from build123d import *

# Parameters (mm, degrees)
CHANFREIN1_SIZE = 0.5


with BuildPart() as part:
    # Esquisse1 → Révolution1 (revolve)
    with BuildSketch(Plane(origin=(0, 0, -20.980989745), x_dir=(-1, 0, 0), z_dir=(0, 0, -1)), mode=Mode.PRIVATE) as r_volution1_sk:
        Polygon((176.591924368, 38.325618202), (176.591924368, 34.825618202), (178.091924368, 34.825618202), (178.091924368, 36.825618202), (181.591924368, 36.825618202), (181.591924368, 38.325618202), align=None)
    revolve(r_volution1_sk.sketch.rotate(Axis((-182.472480167, 39.825618202, -20.980989745), (1, 0, 0)), 270), axis=Axis((-182.472480167, 39.825618202, -20.980989745), (1, 0, 0)))

    # Chanfrein1
    chanfrein1_edges = [part.edges().sort_by_distance(p)[0] for p in [
        (-181.591924368, 39.825618202, -23.980989745),
    ]]
    chamfer(chanfrein1_edges, length=CHANFREIN1_SIZE)


solid = part.part
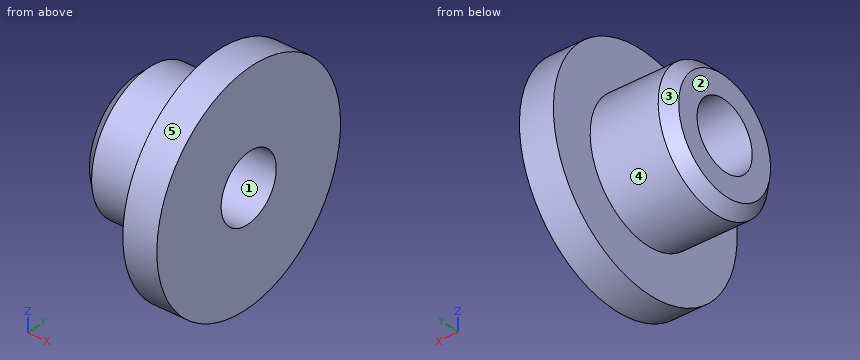
Could you check a few things on this model? Use its own coordinates, in mm. Face numbers are marked on the shaded views. A direction names the side the tool comes from. Coordinates: 2 decimals unless noted, no trailing zeros. Loops run counter-clockwise (first coordinate to the right, second up) from the corner with the lowest first, then second, coordinate; pieces in that order, holes last.
1. Imagine slicing it at A-A (z = -16.75). Please give me the cut outline in (x, y), and give its area (3 significant figures).
2. Imagine slicing it at D-D (z = -24.25). Please give me the cut outline in (x, y), and give its area (4 significant figures).
3. Imagine slicing it at C-C (x = -180.05). Please give me the cut outline in (y, z), and give its area (3 significant figures).
4. Imagine slicing it at B-B (x = -177.85). Please give me the cut outline in (y, z), and give its area (3 significant figures).
5. I need wall thicknesses on L1, parallel to X at y = 38, z = -18.25; L2, parallel to Y at x = -181.3, z = -20.5; L3, parallel to Y at x = -178.5, z = -21.25. Which ranges of each line are inside material? Lowest first, please.
6. We'd pull the mould along Z, two halves only. Please class the marked faces 1, 2 and 3: released by +Z, released by -Z, zero draft, split by the parting line, or undercut.
7. For the marked faces 4 and 5, which set-ups out of +Z, -Z, +X, -X, +Y, -Y let a thin tool reach every point of the face, with its end or its side?
Computed values:
1. outline: (-178.09, 37.16) - (-176.59, 37.16) - (-176.59, 42.49) - (-178.09, 42.49) - close
1. area: 7.99 mm2
2. outline: (-178.09, 36.04) - (-176.59, 36.04) - (-176.59, 43.61) - (-178.09, 43.61) - close
2. area: 11.35 mm2
3. outline: circle Ø6 at (39.83, -20.98); hole circle Ø3 at (39.83, -20.98)
3. area: 21.2 mm2
4. outline: circle Ø10 at (39.83, -20.98); hole circle Ø3 at (39.83, -20.98)
4. area: 71.5 mm2
5. L1: x = -178.09 to -176.59
5. L2: y = 37.08 to 38.4, 41.25 to 42.58
5. L3: y = 36.84 to 38.35, 41.3 to 42.81
6. face 1: undercut
6. face 2: zero draft
6. face 3: split by the parting line
7. face 4: -X
7. face 5: +X, -X
